Input: part model. Units: mm. Frame: model coordinates. A direction names the side the tool comes from. Give positions to 0.01 mm unless a question says otherwise; leave off trailing zeros. Order: outer loops, then holes, each group sorted by start corner. A loop starts at its lowest first (then second) coordinate and runs counter-clockwise, first axis right, second up.
```python
from build123d import *

# Parameters (mm, degrees)
CROQUIS1_W              = 63.5
CROQUIS1_H              = 63.5
CROQUIS1_W_2            = 57.15
CROQUIS1_H_2            = 57.15
SALIENTE_EXTRUIR1_DEPTH = 2400
CROQUIS2_R              = 9.525
CORTAR_EXTRUIR1_DEPTH   = 450
MATRIZL1_COUNT          = 4
MATRIZL1_PITCH          = 410
CROQUIS3_W              = 63.5
CROQUIS3_H              = 90
CORTAR_EXTRUIR2_DEPTH   = 200
CROQUIS4_R              = 7.9375
CORTAR_EXTRUIR3_DEPTH   = 63.5


with BuildPart() as part:
    # Croquis1 → Saliente-Extruir1 (new body)
    with BuildSketch(Plane(origin=(0, 0, 0), x_dir=(1, 0, 0), z_dir=(0, 1, 0))):
        Rectangle(CROQUIS1_W, CROQUIS1_H)
        Rectangle(CROQUIS1_W_2, CROQUIS1_H_2, mode=Mode.SUBTRACT)
    extrude(amount=SALIENTE_EXTRUIR1_DEPTH)

    # Croquis2 → Cortar-Extruir1 (cut)
    with BuildSketch(Plane(origin=(31.75, 0, 0), x_dir=(0, 0, -1), z_dir=(1, 0, 0))):
        with Locations((0, 400)):
            Circle(CROQUIS2_R)
    cortar_extruir1 = extrude(amount=-CORTAR_EXTRUIR1_DEPTH, mode=Mode.SUBTRACT)

    # MatrizL1: Cortar-Extruir1 ×4
    with Locations(*[(0, i * MATRIZL1_PITCH, 0) for i in range(1, MATRIZL1_COUNT)]):
        add(cortar_extruir1, mode=Mode.SUBTRACT)

    # Croquis3 → Cortar-Extruir2 (cut)
    with BuildSketch(Plane.ZY.offset(31.75)):
        with Locations((0, 45)):
            Rectangle(CROQUIS3_W, CROQUIS3_H)
    extrude(amount=-CORTAR_EXTRUIR2_DEPTH, mode=Mode.SUBTRACT)

    # Croquis4 → Cortar-Extruir3 (cut)
    with BuildSketch(Plane.ZY.offset(31.75)):
        with Locations((0, 1860)):
            Circle(CROQUIS4_R)
    extrude(amount=-CORTAR_EXTRUIR3_DEPTH, mode=Mode.SUBTRACT)


solid = part.part
```
1) Cut plane B-B (x = 16). Return the cut outline in (y, z) (3 decimals), then the cut area to 3 significant figures.
2) Line query: probe 1 along Y at (x, z) = (29, 0) (1 decimal); probe 2 along Z at (x, y) = (-30.1, 1630) (3 decimals); probe 3 along Z at (x, y) = (16.5, 916) (3 decimals). Output: solid intervals per line, ascending.
3) Pull-direction query (Z, two-part tool) for faces 1 (the face through (0, 1229, 31.75)), 2 (the face through (0, 1229, -28.575)), 3 (the face through (30, 90, -3)); classes: pulls with the +Z half, pulls with the -Z half, needs draft (parallel to the pull), parting line crosses it, or undercut.
4) Reachability of faces 4 (the face through (-3, 2400, 30)), 5 (the face through (0, 1229, 28.575)) from +Z, -Z, +X, -X, +Y, -Y: full face, straight path, thin tool, end or side. Return the list, or none.
5) Cut plane A-A (y = 360). Return the cut outline in (x, z) (3 decimals).
Geometry says:
1. outline: (90, -31.75) - (2400, -31.75) - (2400, -28.575) - (90, -28.575) - close; (90, 28.575) - (2400, 28.575) - (2400, 31.75) - (90, 31.75) - close
1. area: 14,700 mm2
2. probe 1: y = 90 to 390.5, 409.5 to 800.5, 819.5 to 1210.5, 1229.5 to 1620.5, 1639.5 to 1852.1, 1867.9 to 2400
2. probe 2: z = -31.75 to -9.525, 9.525 to 31.75
2. probe 3: z = -31.75 to -28.575, 28.575 to 31.75
3. face 1: pulls with the +Z half
3. face 2: undercut
3. face 3: needs draft
4. face 4: +Z, -Z, +X, -X, +Y
4. face 5: +Y, -Y
5. outline: (-31.75, -31.75) - (31.75, -31.75) - (31.75, 31.75) - (-31.75, 31.75) - close; hole (-28.575, -28.575) - (28.575, -28.575) - (28.575, 28.575) - (-28.575, 28.575) - close
